from build123d import *

# Parameters (mm, degrees)
SKIZZE1_W                          = 33.6
SKIZZE1_H                          = 32
AUFSATZ_LINEAR_AUSTRAGEN1_DEPTH    = 13
SKIZZE17_W                         = 20
SKIZZE17_H                         = 30
SCHNITT_LINEAR_AUSTRAGEN2_DEPTH    = 6
KERNLOCH_F_R_M2_GEWINDE1_D         = 1.6
VERRUNDUNG2_R                      = 2
DURCHGANGSLOCH_F_R_M52_D           = 5.3
F_3_0MM_CLEARANCE_STIFTLOCH1_D     = 3
F_3_0MM_CLEARANCE_STIFTLOCH1_DEPTH = 5
F_3_0MM_CLEARANCE_STIFTLOCH1_TIP   = 0.901290929
KERNLOCH_F_R_M5_GEWINDE1_D         = 4.2
SKIZZE27_W                         = 33.6
SKIZZE27_H                         = 21.1
SCHNITT_LINEAR_AUSTRAGEN3_DEPTH    = 3
FASE1_SIZE                         = 2
VERRUNDUNG3_R                      = 1


with BuildPart() as part:
    # Skizze1 → Aufsatz-Linear austragen1 (new body)
    with BuildSketch(Plane(origin=(0, 0, 0), x_dir=(1, 0, 0), z_dir=(0, 1, 0))):
        Rectangle(SKIZZE1_W, SKIZZE1_H)
    extrude(amount=AUFSATZ_LINEAR_AUSTRAGEN1_DEPTH)

    # Skizze17 → Schnitt-Linear austragen2 (cut)
    with BuildSketch(Plane(origin=(0, 13, 0), x_dir=(1, 0, 0), z_dir=(0, 1, 0))):
        Rectangle(SKIZZE17_W, SKIZZE17_H)
    extrude(amount=-SCHNITT_LINEAR_AUSTRAGEN2_DEPTH, mode=Mode.SUBTRACT)

    # Kernloch für M2 Gewinde1 (through all)
    with Locations(Plane(origin=(0, 13, 0), x_dir=(1, 0, 0), z_dir=(0, 1, 0))):
        with Locations((-13.75, 13), (13.75, 13), (13.75, -13), (-13.75, -13)):
            Hole(KERNLOCH_F_R_M2_GEWINDE1_D / 2)

    # Verrundung2
    verrundung2_edges = [part.edges().sort_by_distance(p)[0] for p in [
        (-10, 10, 15),
        (-10, 10, -15),
        (10, 10, -15),
        (10, 10, 15),
    ]]
    fillet(verrundung2_edges, radius=VERRUNDUNG2_R)

    # Durchgangsloch für M52 (through all)
    with Locations(Plane(origin=(0, 7, 0), x_dir=(1, 0, 0), z_dir=(0, 1, 0))):
        with Locations((0, 0)):
            Hole(DURCHGANGSLOCH_F_R_M52_D / 2)

    # Ø3.0mm Clearance Stiftloch1
    with Locations(Plane(origin=(0, 0, 0), x_dir=(-1, 0, 0), z_dir=(0, -1, 0))):
        with Locations((-9.5, 0)):
            Hole(F_3_0MM_CLEARANCE_STIFTLOCH1_D / 2, depth=F_3_0MM_CLEARANCE_STIFTLOCH1_DEPTH)
            with Locations((0, 0, -(F_3_0MM_CLEARANCE_STIFTLOCH1_DEPTH + F_3_0MM_CLEARANCE_STIFTLOCH1_TIP / 2))):  # 118° drill point
                Cone(0, F_3_0MM_CLEARANCE_STIFTLOCH1_D / 2, F_3_0MM_CLEARANCE_STIFTLOCH1_TIP, mode=Mode.SUBTRACT)

    # Kernloch für M5 Gewinde1 (through all)
    with Locations(Plane(origin=(0, 0, 0), x_dir=(-1, 0, 0), z_dir=(0, -1, 0))):
        with Locations((0, -11)):
            Hole(KERNLOCH_F_R_M5_GEWINDE1_D / 2)

    # Skizze27 → Schnitt-Linear austragen3 (cut)
    with BuildSketch(Plane.XZ):
        with Locations((0, 5.45)):
            Rectangle(SKIZZE27_W, SKIZZE27_H)
    extrude(amount=-SCHNITT_LINEAR_AUSTRAGEN3_DEPTH, mode=Mode.SUBTRACT)

    # Fase1
    fase1_edges = [part.edges().sort_by_distance(p)[0] for p in [
        (-16.8, 6.5, -16),
        (16.8, 6.5, -16),
        (16.8, 8, 16),
        (-16.8, 8, 16),
    ]]
    chamfer(fase1_edges, length=FASE1_SIZE)

    # Verrundung3
    verrundung3_edges = [part.edges().sort_by_distance(p)[0] for p in [
        (0, 3, 16),
        (-16.8, 3, 4.45),
        (15.8, 3, 15),
        (-15.8, 3, 15),
        (-16.8, 0, -9.55),
        (0, 0, -16),
        (-15.8, 0, -15),
        (15.8, 0, -15),
        (16.8, 0, -9.55),
        (16.8, 3, 4.45),
    ]]
    fillet(verrundung3_edges, radius=VERRUNDUNG3_R)


solid = part.part
Read the model definition and answer for the solid it produces. Units are mm, in the model's axes. A direction names the side the tool comes from. Give positions to 0.01 mm unless a question says otherwise; leave off trailing zeros. Write each loop counter-clockwise with the first axis right and the second up, starting at its lowest first coordinate (ties: lowest second). Pieces come first, ordered by that corner, then holes. Notation, with made-up numbers: (83, 67) - (142, 67) arc R7 ccw to (142, 76) - close; hole circle Ø9 at (87, 38.5). An arc over 180 degrees is marked (long way). Answer in a Markdown table with one row per item. Add a question column.
Item 1: Section C-C, the plane y = 8.25 is taken. Write down the section's boundary in (x, z).
Item 2: Find the intervals of material crossed by L1, parallel to X at y = 5.75, z = -13; L2, parallel to Z at x = 0, y = 3.9; L3, parallel to Z at x = -13.75, y = 10, in increasing order.
Item 3: Flat-ended cylindrical pins translate along their axes: P1, Ø1.3, axis at x = 13.75, z = -13, coming from the +Y side; P2, Ø6, axis at x = 4.5, z = 5.5, coming from the -Y side; P3, Ø5, axis at y = 2, z = 8, coming from the +X side. Find the tip coordinate at first contact, or state that the pin passes through.
Item 4: A tool of negligible diameter and unlimited length cuts with its end or side. For faces 5 (the face through (10, 10, 0)), 6 (the face through (0, 8, 16)), from which of +Z, -Z, +X, -X, +Y, -Y can it reach the whole face along a straight path? Write none if from no direction.
Item 5: Determine the mould class of faces 1 (the face through (9.4, 9.96, 14.43)), 2 (the face through (15.612, 0.301, -14.784)), 3 (the face through (-15.8, 6.9, -15)), 4 (the face through (9.707, 5.745, 0.159)) for opening direction X: pulls with the +X half, pulls with the -X half, needs draft (parallel to the pull), parting line crosses it, or undercut.
Item 6: Section A-A, the plane x = -13.75 is taken. Write down the section's boundary in (y, z).
Item 7: Section B-B, the plane y = 2.5 is taken. Write down the section's boundary in (x, z).
Item 8: Section D-D, the plane z = 5.5 is taken. Write down the section's boundary in (x, y).
Recorded:
| question | item | result |
|---|---|---|
| 1 | outline | (-16.8, -14) - (-14.8, -16) - (14.8, -16) - (16.8, -14) - (16.8, 14) - (14.8, 16) - (-14.8, 16) - (-16.8, 14) - close; hole circle Ø1.6 at (-13.75, -13); hole circle Ø1.6 at (-13.75, 13); hole (-10, -13) arc R2 ccw to (-8, -15) - (8, -15) arc R2 ccw to (10, -13) - (10, 13) arc R2 ccw to (8, 15) - (-8, 15) arc R2 ccw to (-10, 13) - close; hole circle Ø1.6 at (13.75, -13); hole circle Ø1.6 at (13.75, 13) |
| 2 | L1 | x = -16.8 to -14.55, -12.95 to 12.95, 14.55 to 16.8 |
| 2 | L2 | z = -16 to -2.65, 2.65 to 8.9, 13.1 to 15.99 |
| 2 | L3 | z = -16 to -13.8, -12.2 to 12.2, 13.8 to 16 |
| 3 | P1 | passes through |
| 3 | P2 | stops at y = 3 |
| 3 | P3 | stops at x = 16.8 |
| 4 | face 5 | +Y |
| 4 | face 6 | +Z, +X, -X, +Y, -Y |
| 5 | face 1 | undercut |
| 5 | face 2 | pulls with the +X half |
| 5 | face 3 | pulls with the -X half |
| 5 | face 4 | undercut |
| 6 | outline | (0, -15) arc R1 ccw to (1, -16) - (13, -16) - (13, -13.8) - (0, -13.8) - close; (0, -12.2) - (13, -12.2) - (13, 12.2) - (3, 12.2) - (3, -5.1) - (0, -5.1) - close; (3, 13.8) - (13, 13.8) - (13, 16) - (4, 16) arc R1 ccw to (3, 15) - close |
| 7 | outline | (-16.8, -14) - (-14.8, -16) - (14.8, -16) - (16.8, -14) - (16.8, -5.1) - (-16.8, -5.1) - close; hole circle Ø1.6 at (-13.75, -13); hole circle Ø1.6 at (13.75, -13) |
| 8 | outline | (-16.8, 4) arc R1 ccw to (-15.8, 3) - (15.8, 3) arc R1 ccw to (16.8, 4) - (16.8, 13) - (10, 13) - (10, 7) - (-10, 7) - (-10, 13) - (-16.8, 13) - close |
